Build history of the part. All positions in model axes, mm. A direction names the side the tool comes from. Give positions to 0.01 mm unless a question says otherwise; leave off trailing zeros. Loops run counter-clockwise (first coordinate to the right, second up) from the corner with the lowest first, then second, coordinate; pieces in that order, holes last. Notation, with made-up numbers: (68.25, 11.25) -> (89.25, 11.25) arc R7 ccw to (89.25, 17.25) -> close; hole circle Ø9 at (10, -14.5). An arc over 180 degrees is marked (long way). Answer as a JSON object with one key per item and string values. Group by question number.
from build123d import *

# Parameters (mm, degrees)
SKETCH1_W           = 150
SKETCH1_H           = 200
BOSS_EXTRUDE1_DEPTH = 100
SHELL2_T            = -5
SKETCH5_R           = 1.9
CUT_EXTRUDE2_DEPTH  = 10
BOSS_EXTRUDE4_DEPTH = 200
SKETCH9_W           = 101.133931545
SKETCH9_H           = 31.996148617
CUT_EXTRUDE4_DEPTH  = 236.849528301
SKETCH10_R          = 4
CUT_EXTRUDE5_DEPTH  = 10
CUT_EXTRUDE7_REACH  = 162.078
SKETCH11_W          = 140
SKETCH11_H          = 5
SKETCH15_R          = 1.2
CUT_EXTRUDE11_DEPTH = 10
SKETCH36_W          = 60
SKETCH36_H          = 5
BOSS_EXTRUDE7_DEPTH = 10
SKETCH37_R          = 3.5
CUT_EXTRUDE15_DEPTH = 60
SKETCH38_R          = 5
CUT_EXTRUDE16_DEPTH = 70
SKETCH40_W          = 179.165652401
SKETCH40_H          = 85.135231114
SKETCH40_W_2        = 87.941982163
SKETCH40_H_2        = 17
CUT_EXTRUDE18_DEPTH = 236.849528301
FILLET1_R           = 2


with BuildPart() as part:
    # Sketch1 → Boss-Extrude1 (new body)
    with BuildSketch(Plane(origin=(0, 0, 0), x_dir=(1, 0, 0), z_dir=(0, 1, 0))):
        Rectangle(SKETCH1_W, SKETCH1_H)
    extrude(amount=BOSS_EXTRUDE1_DEPTH)

    # Shell2
    shell2_openings = [part.faces().sort_by_distance(p)[0] for p in [
        (0, 50, -100),
        (0, 50, 100),
    ]]
    offset(amount=SHELL2_T, openings=shell2_openings, kind=Kind.INTERSECTION)

    # Sketch5 → Cut-Extrude2 (cut)
    with BuildSketch(Plane.XZ):
        with Locations(Location((-65, 91, 0), (0, 0, 270))):
            Circle(SKETCH5_R)
        with Locations(Location((-35, 91, 0), (0, 0, 270))):
            Circle(SKETCH5_R)
        with Locations(Location((-65, 67, 0), (0, 0, 270))):
            Circle(SKETCH5_R)
        with Locations(Location((-35, 67, 0), (0, 0, 270))):
            Circle(SKETCH5_R)
    cut_extrude2 = extrude(amount=-CUT_EXTRUDE2_DEPTH, mode=Mode.SUBTRACT)

    # Mirror2: Cut-Extrude2 across plane
    add(cut_extrude2.mirror(Plane.XY), mode=Mode.SUBTRACT)

    # Sketch8 → Boss-Extrude4 (add, through all)
    with BuildSketch(Plane.XY.offset(100)):
        Polygon((-15, 17), (75, 17), (75, 22), (-20, 22), (-20, 0), (-15, 0), align=None)
    extrude(amount=-BOSS_EXTRUDE4_DEPTH)

    # Sketch9 → Cut-Extrude4 (cut, through all)
    with BuildSketch(Plane.XY.offset(100)):
        with Locations((35.566965773, 1.001925691)):
            Rectangle(SKETCH9_W, SKETCH9_H)
    extrude(amount=-CUT_EXTRUDE4_DEPTH, mode=Mode.SUBTRACT)

    # Sketch10 → Cut-Extrude5 (cut)
    with BuildSketch(Plane.XZ.offset(-17)):
        with Locations((60, 0)):
            Circle(SKETCH10_R)
    extrude(amount=-CUT_EXTRUDE5_DEPTH, mode=Mode.SUBTRACT)

    # Cut-Extrude7: up to this face of the body (flat: up to its plane)
    cut_extrude7_end = Plane(part.part.faces().sort_by_distance((-44.954220044, 5, 0))[0])
    # Sketch11 → Cut-Extrude7 (cut, up to the picked face)
    with BuildSketch(Plane(origin=(0, 100, 0), x_dir=(1, 0, 0), z_dir=(0, 1, 0)), mode=Mode.PRIVATE) as cut_extrude7_sk1:
        with Locations((0, -92.5)):
            Rectangle(SKETCH11_W, SKETCH11_H)
    cut_extrude7_tool1 = split(extrude(cut_extrude7_sk1.sketch, amount=-CUT_EXTRUDE7_REACH, mode=Mode.PRIVATE), bisect_by=cut_extrude7_end, keep=Keep.BOTH, mode=Mode.PRIVATE)
    cut_extrude7 = cut_extrude7_tool1.solids().sort_by(Axis((0, 100, 92.5), (0, -1, 0)))[0]
    add(cut_extrude7, mode=Mode.SUBTRACT)

    # Mirror3: Cut-Extrude7 across plane
    add(cut_extrude7.mirror(Plane.XY), mode=Mode.SUBTRACT)

    # Sketch15 → Cut-Extrude11 (cut)
    with BuildSketch(Plane(origin=(0, 100, 0), x_dir=(1, 0, 0), z_dir=(0, 1, 0))):
        with Locations(Location((50, 28, 0), (0, 0, 270))):
            Circle(SKETCH15_R)
        with Locations(Location((50, -28, 0), (0, 0, 270))):
            Circle(SKETCH15_R)
        with Locations(Location((-20, 20, 0), (0, 0, 270))):
            Circle(SKETCH15_R)
        with Locations(Location((-20, -20, 0), (0, 0, 270))):
            Circle(SKETCH15_R)
    extrude(amount=-CUT_EXTRUDE11_DEPTH, mode=Mode.SUBTRACT)

    # Sketch36 → Boss-Extrude7 (add)
    with BuildSketch(Plane.ZY.offset(-70)):
        with Locations((-13.202053215, 62.5)):
            Rectangle(SKETCH36_W, SKETCH36_H)
    boss_extrude7 = extrude(amount=BOSS_EXTRUDE7_DEPTH)

    # Mirror5: Boss-Extrude7 across plane
    add(boss_extrude7.mirror(Plane(origin=(0, 0, 0), x_dir=(0, 0, 1), z_dir=(1, 0, 0))))

    # Sketch37 → Cut-Extrude15 (cut)
    with BuildSketch(Plane(origin=(75, 0, 0), x_dir=(0, 0, -1), z_dir=(1, 0, 0))):
        with Locations((0, 75)):
            Circle(SKETCH37_R)
    extrude(amount=-CUT_EXTRUDE15_DEPTH, mode=Mode.SUBTRACT)

    # Sketch38 → Cut-Extrude16 (cut)
    with BuildSketch(Plane.ZY.offset(75)):
        with Locations((0, 80)):
            Circle(SKETCH38_R)
    extrude(amount=-CUT_EXTRUDE16_DEPTH, mode=Mode.SUBTRACT)

    # Sketch40 → Cut-Extrude18 (cut, through all)
    with BuildSketch(Plane.XY.offset(100)):
        with Locations((-9.51631739, 64.567615557)):
            Rectangle(SKETCH40_W, SKETCH40_H)
        with Locations((-63.970991082, 13.5)):
            Rectangle(SKETCH40_W_2, SKETCH40_H_2)
    extrude(amount=-CUT_EXTRUDE18_DEPTH, mode=Mode.SUBTRACT)

    # Fillet1
    fillet1_edges = [part.edges().sort_by_distance(p)[0] for p in [
        (-15, 0, 0),
        (-20, 5, 0),
        (-15, 17, 0),
    ]]
    fillet(fillet1_edges, radius=FILLET1_R)


solid = part.part
(1) Pin check, flat tips, straight feed: pin 1 (8 mm diameter, centred on y = 17, z = 57.5, fed in from -X); pin 2 (5 mm diameter, centred on x = 29, y = 13.5, fed in from +Z); pin 3 (2.5 mm diameter, centred on y = 20.5, z = -92, fed in from -X); pin 4 (12 mm diameter, centred on y = 9, z = 39, fed in from +X). Stop position of each tip, or through.
(2) 3-axis set-ups, long thin cutter, end or side, ignore diameter. For faces 1 (the flat face through (70, 20, -93)), 2 (the flat face through (0, 18, -100)), 3 (the flat face through (14.4, 17.4, -95)): which of +Z, -Z, +X, -X, +Y, -Y reach the whole face in a straight line?
(3) Saw through at D-D on x = -58.5. List the corners of the cut face in (y, z).
(4) Saw through at B-B on x = 60. List the corners of the cut face in (y, z), plus the area to 3 significant figures.
(5) Pull direction X, two halves, no side cores. Call faces 4 (the flat face through (75, 19, 1)), 5 (the cylindrical face through (-66.855, 2.465, -67.412)), 6 (the cylindrical face through (-36.156, 2.465, -68.508)), 7 (the flat face through (70, 20, 92)): pulls with the +X half, pulls with the -X half, needs draft (parallel to the pull), parting line crosses it, or undercut.
(6) Probe line 1 along Z through (x, y) = (60, 18.2); line 2 along Z through (x, y) = (44.5, 19); line 3 along X through (y, z) = (4.05, 91). List the from-to ranges inside material, lowest first. Write a range as [from, to].
(7) Saw through at A-A on x = 4.5. List the corners of the cut face in (y, z).
(8) Saw through at C-C on z = 78.5. List the corners of the cut face in (x, y).
Calculated:
{
 "1": {"pin 1": "stops at x = -20", "pin 2": "passes through", "pin 3": "stops at x = 70", "pin 4": "stops at x = -15"},
 "2": {"face 1": "-X, +Y, -Y", "face 2": "-Z, +X, -X, +Y, -Y", "face 3": "-X, +Y"},
 "3": {"outline": "(0, -100) -> (5, -100) -> (5, 100) -> (0, 100) -> close"},
 "4": {"outline": "(17, -100) -> (22, -100) -> (22, -95) -> (17, -95) -> close; (17, -90) -> (22, -90) -> (22, -4) -> (17, -4) -> close; (17, 4) -> (22, 4) -> (22, 90) -> (17, 90) -> close; (17, 95) -> (22, 95) -> (22, 100) -> (17, 100) -> close", "area": "910 mm^2"},
 "5": {"face 4": "pulls with the +X half", "face 5": "undercut", "face 6": "undercut", "face 7": "pulls with the -X half"},
 "6": {"line 1": "z = [-100, -95], [-90, -4], [4, 90], [95, 100]", "line 2": "z = [-100, -95], [-90, 90], [95, 100]", "line 3": "x = [-75, -66.9], [-63.1, -36.9], [-33.1, -15]"},
 "7": {"outline": "(17, -100) -> (22, -100) -> (22, -95) -> (17, -95) -> close; (17, -90) -> (22, -90) -> (22, 90) -> (17, 90) -> close; (17, 95) -> (22, 95) -> (22, 100) -> (17, 100) -> close"},
 "8": {"outline": "(-75, 0) -> (-17, 0) arc R2 ccw to (-15, 2) -> (-15, 15) arc R2 cw to (-13, 17) -> (75, 17) -> (75, 22) -> (-20, 22) -> (-20, 7) arc R2 cw to (-22, 5) -> (-75, 5) -> close"}
}
